The listing builds one solid part. Answer for the finished solid, in the listing's coordinates (mm). A direction names the side the tool comes from. Coordinates: 2 decimals unless noted, no trailing zeros. Order: outer loops, then holes, each group sorted by start corner. A loop starts at its lowest first (then second) coordinate and runs counter-clockwise, first axis right, second up. Notation, with made-up numbers: (25.25, 6) -> (81.25, 6) arc R34 cw to (81.25, 40) -> close; hole circle Ø1 at (17.25, 79). An arc over 180 degrees is marked (long way). Answer in a Markdown table with one row per item.
```python
from build123d import *

# Parameters (mm, degrees)
F0_R     = 2.7
F0_R_2   = 1.5
F1_DEPTH = 5
F2_DEPTH = 2.8


with BuildPart() as f1:
    # F0 (on Front) → F1 (new body)
    with BuildSketch(Plane.XZ):
        with Locations((23.7, -0.8)):
            Circle(F0_R)
        with Locations((23.7, -0.8)):
            Circle(F0_R_2, mode=Mode.SUBTRACT)
    extrude(amount=F1_DEPTH)



with BuildPart() as f1b:
    # F0 (on Front) → F1, piece 2 (new body)
    with BuildSketch(Plane.XZ):
        with Locations((9.7, -0.8)):
            Circle(F0_R)
        with Locations((9.7, -0.8)):
            Circle(F0_R_2, mode=Mode.SUBTRACT)
    extrude(amount=F1_DEPTH)


with BuildPart() as f1_1:
    add(f1.part)

    add(f1b.part)  # F2 merges F1b
    # F0 (on Front) → F2 (join)
    with BuildSketch(Plane.XZ):
        with BuildLine():
            Line((11.9999478371, -24), (32, -24))
            Line((32, -24), (32, 24))
            Line((32, 24), (-32, 24))
            Line((-32, 24), (-32, -24))
            Line((-32, -24), (-11.9996363419, -24))
            Line((-11.9996363419, -24), (-11.9996363419, -27.906578041))
            ThreePointArc((-11.9996363419, -27.906578041), (-0.0644023145, -39.9998271797), (11.9999478371, -28.0353822933))
            ThreePointArc((11.9999478371, -28.0353822933), (12, -28), (11.9999478371, -27.9646177067))
            Line((11.9999478371, -27.9646177067), (11.9999478371, -24))
        make_face()
        with Locations((9.7, -0.8)):
            Circle(F0_R, mode=Mode.SUBTRACT)
        with Locations((23.7, -0.8)):
            Circle(F0_R, mode=Mode.SUBTRACT)
        with Locations((9.7, -0.8)):
            Circle(F0_R)
        with Locations((9.7, -0.8)):
            Circle(F0_R_2, mode=Mode.SUBTRACT)
        with Locations((9.7, -0.8)):
            Circle(F0_R_2)
        with Locations((23.7, -0.8)):
            Circle(F0_R)
        with Locations((23.7, -0.8)):
            Circle(F0_R_2, mode=Mode.SUBTRACT)
        with Locations((23.7, -0.8)):
            Circle(F0_R_2)
    extrude(amount=-F2_DEPTH)


solid = f1_1.part
```
(1) Flat-ended cylindrical pins translate along their axes: pin 1 (1 mm diameter, centred on x = 25.5, y = -1.5, fed in from +Z); pin 2 (2 mm diameter, centred on x = -23.5, y = 1.5, fed in from -Z); pin 3 (1.5 mm diameter, centred on x = -1.5, z = 10, fed in from -Y). Find the tip coordinate at first contact, or state that the pin passes through.
Check values:
| item | result |
|---|---|
| pin 1 | z = 1.57 |
| pin 2 | z = -24 |
| pin 3 | y = 0 |
(2) For a pull along X with two mould halves and no side action, classify faces 1 (the flat face through (-22, 1, -24)), 2 (the cylindrical face through (11.086, -2.465, -1.375)), 3 (the flat face through (12, 1, -26)) as released by +X, released by -X, zero draft, split by the parting line, or undercut.
Check values:
| item | result |
|---|---|
| face 1 | zero draft |
| face 2 | undercut |
| face 3 | released by +X |
(3) Which of the six approach directions +Z, -Z, +X, -X, +Y, -Y give full straight-line access (tool end or side, diameter ignored) to faces 4 (the flat face through (-12, 1, -26)), 5 (the flat face through (22, 1, -24)), 6 (the cylindrical face through (21, -2.5, -0.7))?
Check values:
| item | result |
|---|---|
| face 4 | -Z, -X, +Y, -Y |
| face 5 | -Z, +X, +Y, -Y |
| face 6 | -Y |
(4) A cutting plane is placed at B-B, the plane z = -0.8. Determine the outline of the cut face in (x, y).
Check values:
| item | result |
|---|---|
| outline | (-32, 0) -> (7, 0) -> (7, -5) -> (8.2, -5) -> (8.2, 0) -> (11.2, 0) -> (11.2, -5) -> (12.4, -5) -> (12.4, 0) -> (21, 0) -> (21, -5) -> (22.2, -5) -> (22.2, 0) -> (25.2, 0) -> (25.2, -5) -> (26.4, -5) -> (26.4, 0) -> (32, 0) -> (32, 2.8) -> (-32, 2.8) -> close |
(5) A cutting plane is placed at C-C, the plane x = 23.7. Determine the outline of the cut face in (y, z), then the cut area to 3 significant figures.
Check values:
| item | result |
|---|---|
| outline | (-5, -3.5) -> (0, -3.5) -> (0, -24) -> (2.8, -24) -> (2.8, 24) -> (0, 24) -> (0, 1.9) -> (-5, 1.9) -> (-5, 0.7) -> (0, 0.7) -> (0, -2.3) -> (-5, -2.3) -> close |
| area | 146 mm² |
(6) A cutting plane is placed at A-A, the plane y = 1. Determine the outline of the cut face in (x, z), then the cut area to 3 significant figures.
Check values:
| item | result |
|---|---|
| outline | (-32, -24) -> (-12, -24) -> (-12, -27.91) arc R12 ccw to (12, -28.04) arc R12 ccw to (12, -27.96) -> (12, -24) -> (32, -24) -> (32, 24) -> (-32, 24) -> close |
| area | 3,390 mm² |
(7) A cutting plane is placed at D-D, the plane x = 9.7. Determine the outline of the cut face in (y, z), then the cut area to 3 significant figures.
Check values:
| item | result |
|---|---|
| outline | (-5, -3.5) -> (0, -3.5) -> (0, -35.06) -> (2.8, -35.06) -> (2.8, 24) -> (0, 24) -> (0, 1.9) -> (-5, 1.9) -> (-5, 0.7) -> (0, 0.7) -> (0, -2.3) -> (-5, -2.3) -> close |
| area | 177 mm² |
(8) Find the intervals of material crossed by line 1 along Z through (x, y) = (9.7, -3.65); line 2 along Y through (x, z) = (11.5, 9); line 3 along Z through (x, y) = (-18.5, 1.5), in increasing order. Write a range as from..to.
Check values:
| item | result |
|---|---|
| line 1 | -3.5..-2.3, 0.7..1.9 |
| line 2 | 0..2.8 |
| line 3 | -24..24 |
